The model under review builds one solid part; all positions refer to its coordinate system, in mm. Coordinates: 2 decimals unless noted, no trailing zeros. Loops run counter-clockwise (first coordinate to the right, second up) from the corner with the lowest first, then second, coordinate; pieces in that order, holes last. Notation, with made-up numbers: (-35.5, -23.5) - (-25.5, -23.5) arc R36 cw to (-25.5, 14.5) - close; hole circle Ø5 at (5, -3.5). An arc over 180 degrees is marked (long way). Answer in a Markdown table with one row per item. Add a question column.
(1) For P1, Ø1, axis at y = -41.5, z = 3, coming from the +X side; P2, Ø1, axis at y = -56, z = 1, coming from the -X side; P3, Ø1.5, axis at y = -66, z = 2, coming from the -X side, all flat-tipped, find the tip position at first contact; note any pin that passes through.
(2) Mouldability with a two-part tool opening along Y and no side actions: class faces 1 (the flat face through (-71.425, 11, 2)), 2 (the cylindrical face through (-2.95, -32.87, 2.03)), 3 (the cylindrical face through (-65.42, 5.86, 1.97)), 4 (the flat face through (8.855, -36.429, 1.972)) as +Y half, -Y half, draft (parallel to the pull), parting line (faces both ways), or undercut.
(3) For line 1 along X through (y, z) = (8, 1.55) (3 decimals); line 2 along X through (y, z) = (3.5, 1.8); line 3 along Y through (x, z) = (-28.5, 2.1), list the stretches that pass through material, from the lowest coordinate up.
(4) We need section D-D on y = 3. Write out the cut boundary in (x, z), plus the area to 3 significant figures.
(5) We need section A-A on y = -16.5. Write out the cut boundary in (x, z).
(6) We need section B-B on x = -60. Write out the cut boundary in (y, z).
(7) We need section C-C on z = 0.7. Write out the cut boundary in (x, y) (3 decimals), plus the area to 3 significant figures.
from build123d import *

# Parameters (mm, degrees)
SKETCH1_R           = 4
BOSS_EXTRUDE1_DEPTH = 4
SKETCH2_R           = 20
CUT_EXTRUDE1_DEPTH  = 10


with BuildPart() as part:
    # Sketch1 → Boss-Extrude1 (new body)
    with BuildSketch(Plane.XY):
        Polygon((-71.425004503, 17.68546584), (28.574995497, 17.68546584), (28.574995497, 5.27207622), (-11.425004503, -79.31453416), (-31.425004503, -79.31453416), (-71.425004503, 5.27207622), align=None)
        with Locations((-61.425004503, 5.68546584)):
            Circle(SKETCH1_R, mode=Mode.SUBTRACT)
        with Locations((18.574995497, 5.68546584)):
            Circle(SKETCH1_R, mode=Mode.SUBTRACT)
        with Locations((-21.425004503, -67.31453416)):
            Circle(SKETCH1_R, mode=Mode.SUBTRACT)
    extrude(amount=BOSS_EXTRUDE1_DEPTH)

    # Sketch2 → Cut-Extrude1 (cut)
    with BuildSketch(Plane.XY.offset(4)):
        with Locations((-21.425004503, -25.21253416)):
            Circle(SKETCH2_R)
    extrude(amount=-CUT_EXTRUDE1_DEPTH, mode=Mode.SUBTRACT)


solid = part.part
Outcome:
| question | item | result |
|---|---|---|
| 1 | P1 | x = 6.69 |
| 1 | P2 | x = -42.69 |
| 1 | P3 | x = -38.08 |
| 2 | face 1 | draft |
| 2 | face 2 | undercut |
| 2 | face 3 | undercut |
| 2 | face 4 | -Y half |
| 3 | line 1 | -71.425 to -64.687, -58.163 to 15.313, 21.837 to 28.575 |
| 3 | line 2 | -70.59 to -64.78, -58.07 to 15.22, 21.93 to 27.74 |
| 3 | line 3 | -79.31 to -43.92, -6.51 to 17.69 |
| 4 | outline | (-70.35, 0) - (-64.39, 0) - (-64.39, 4) - (-70.35, 4) - close; (-58.46, 0) - (15.61, 0) - (15.61, 4) - (-58.46, 4) - close; (21.54, 0) - (27.5, 0) - (27.5, 4) - (21.54, 4) - close |
| 4 | area | 344 mm² |
| 5 | outline | (-61.13, 0) - (-39.43, 0) - (-39.43, 4) - (-61.13, 4) - close; (-3.42, 0) - (18.28, 0) - (18.28, 4) - (-3.42, 4) - close |
| 6 | outline | (-18.89, 0) - (1.95, 0) - (1.95, 4) - (-18.89, 4) - close; (9.42, 0) - (17.69, 0) - (17.69, 4) - (9.42, 4) - close |
| 7 | outline | (-71.425, 5.272) - (-31.425, -79.315) - (-11.425, -79.315) - (28.575, 5.272) - (28.575, 17.685) - (-71.425, 17.685) - close; hole circle Ø8 at (-61.425, 5.685); hole circle Ø40 at (-21.425, -25.213); hole circle Ø8 at (-21.425, -67.315); hole circle Ø8 at (18.575, 5.685) |
| 7 | area | 4,910 mm² |
